from build123d import *

# Parameters (mm, degrees)
F3_W       = 12
F3_H       = 40
F4_DEPTH   = 4
F5_R       = 2
F6_R       = 0.9
F7_DEPTH   = 11.5
F8_SIZE2   = 2.4727296775
F8_SIZE    = 0.9
F8_2_SIZE2 = 2.4727296775
F8_2_SIZE  = 0.9


with BuildPart() as f4:
    # F3 (on Top) → F4 (new body)
    with BuildSketch(Plane.XY):
        Rectangle(F3_W, F3_H)
    extrude(amount=F4_DEPTH)

    # F5
    f5_edges = [f4.edges().sort_by_distance(p)[0] for p in [
        (6, 0, 4),
        (-6, 0, 4),
        (0, -20, 4),
        (6, -20, 2),
        (-6, 20, 2),
        (6, 20, 2),
        (0, 20, 4),
        (-6, -20, 2),
    ]]
    fillet(f5_edges, radius=F5_R)

    # F6 (on face) → F7 (join)
    with BuildSketch(Plane(origin=(0, 0, 0), x_dir=(1, 0, 0), z_dir=(0, 0, -1))):
        with Locations((0, -16)):
            Circle(F6_R)
        with Locations((0, 16)):
            Circle(F6_R)
    extrude(amount=F7_DEPTH)

    # F8
    f8_edges = [f4.edges().sort_by_distance(p)[0] for p in [
        (-0.9, 16, -11.5),
    ]]
    f8_side = f4.faces().sort_by_distance((0, 16, -11.5))[0]
    chamfer(f8_edges, length=F8_SIZE, length2=F8_SIZE2, reference=f8_side)

    # F8#2
    f8_2_edges = [f4.edges().sort_by_distance(p)[0] for p in [
        (-0.9, -16, -11.5),
    ]]
    f8_2_side = f4.faces().sort_by_distance((0, -16, -11.5))[0]
    chamfer(f8_2_edges, length=F8_2_SIZE, length2=F8_2_SIZE2, reference=f8_2_side)


solid = f4.part
Part model, mm, in its own coordinate system. A direction names the side the tool comes from. Coordinates: 2 decimals unless noted, no trailing zeros. Loops run counter-clockwise (first coordinate to the right, second up) from the corner with the lowest first, then second, coordinate; pieces in that order, holes last. Notation, with made-up numbers: M 77,9 L 105,9 A33 ccw 105,43 Z; hole C 68.25,60 d1. An arc over 180 degrees is marked long. Use a Markdown table: item, result. Add a question column.
Q1. Cut at B-B (x = 2.75). Write the cut outline in (y, z), and give its area (3 significant figures).
Q2. Pin check, flat tips, straight feed: P1, Ø4, axis at x = 1, z = -7.5, coming from the -Y side; P2, Ø3.5, axis at x = 0, y = 1, coming from the -Z side. Stop position of each tip, or through.
Q3. Mould opens along Y. For faces 1 (the flat face through (-6, 0, 1)), 2 (the conical face through (-0.046, -16.353, -10.521)), 3 (the cylindrical face through (-5.43, -19.4, 1.01)), 4 (the flat face through (0, 20, 1)) say: +Y half, -Y half, draft (parallel to the pull), parting line (faces both ways), or undercut.
Q4. Probe L1, parallel to Z at x = 1.25, y = -15.5; L2, parallel to Y at x = 0.25, z = -1; L3, parallel to Y at x = 0.75, z = -3.25. List the from-to ranges inside material, lowest first.
Q5. Which spindle directions (+Z, -Z, +X, -X, +Y, -Y) get a long thin tool onto all of the face, cutting with end or side? Do faces 5 (the cylindrical face through (-5.43, 19.4, 1.01)), 6 (the cylindrical face through (-0.12, 15.11, -4.45)). Say none if no direction does.
Q6. Cut at A-A (z = -0.75). Write the cut outline in (x, y), and give its area (3 significant figures).
Q7. Cut at C-C (y = -8.5). Write the cut outline in (x, z).
Worked out:
| question | item | result |
|---|---|---|
| 1 | outline | M -20,0 L 20,0 L 20,2 A2 ccw 18,4 L -18,4 A2 ccw -20,2 Z |
| 1 | area | 158 mm2 |
| 2 | P1 | stops at y = -16.9 |
| 2 | P2 | stops at z = 0 |
| 3 | face 1 | draft |
| 3 | face 2 | undercut |
| 3 | face 3 | -Y half |
| 3 | face 4 | +Y half |
| 4 | L1 | z = 0 to 4 |
| 4 | L2 | y = -16.86 to -15.14, 15.14 to 16.86 |
| 4 | L3 | y = -16.5 to -15.5, 15.5 to 16.5 |
| 5 | face 5 | +Z, -Z, -X, +Y |
| 5 | face 6 | -Z |
| 6 | outline | C 0,-16 d1.8; C 0,16 d1.8 |
| 6 | area | 5.09 mm2 |
| 7 | outline | M -6,0 L 6,0 L 6,2 A2 ccw 4,4 L -4,4 A2 ccw -6,2 Z |
